Geometry check sheet. Reference: the model listing, model coordinates, mm. Round coordinates to 2 decimals unless told otherwise and drop trailing zeros. Order: outer loops, then holes, each group sorted by start corner. A loop starts at its lowest first (then second) coordinate and runs counter-clockwise, first axis right, second up.
(1) Material ranges on line 1 along Y through (x, z) = (-43, 137.3) (3 decimals); line 2 along Y through (x, z) = (-376, 136.55), recorded low to high.
(2) Sectioned sample at C-C (z = 138.15). Record the boundary of the cut face in (x, y) (3 decimals).
(3) Sectioned sample at A-A (x = -323.5). Record the boundary of the cut face in (y, z) (1 decimal).
Solid Edge part; units mm, degrees
sketch "Sketch1" plane through (0, 0, 135.9785) normal (0, 0, 1) x (1, 0, 0)
  line L0 (35.165, 9) -> (35.165, -373)
  arc A0 (35.165, -373) -> (9, -399.165) centre (9, -373) cw
  line L1 (9, -399.165) -> (-373, -399.165)
  arc A1 (-373, -399.165) -> (-399.165, -373) centre (-373, -373) cw
  line L2 (-399.165, -373) -> (-399.165, 9)
  arc A2 (-399.165, 9) -> (-373, 35.165) centre (-373, 9) cw
  line L3 (-373, 35.165) -> (9, 35.165)
  arc A3 (9, 35.165) -> (35.165, 9) centre (9, 9) cw
  line L4 (33.165, 9) -> (33.165, -373)
  line L5 (9, -397.165) -> (-373, -397.165)
  line L6 (-397.165, -373) -> (-397.165, 9)
  line L7 (-373, 33.165) -> (9, 33.165)
  arc A4 (33.165, -373) -> (9, -397.165) centre (9, -373) cw
  arc A5 (-373, -397.165) -> (-397.165, -373) centre (-373, -373) cw
  arc A6 (-397.165, 9) -> (-373, 33.165) centre (-373, 9) cw
  arc A7 (9, 33.165) -> (33.165, 9) centre (9, 9) cw
extrude "Protrusion1" add sketch "Sketch1" along normal blind 6
properties material "Polyurethene"
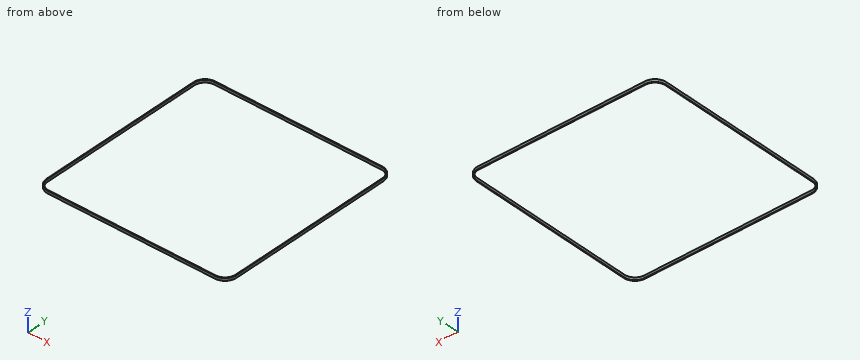
Answer below:
1. line 1: y = -399.165 to -397.165, 33.165 to 35.165
1. line 2: y = -398.99 to -396.98, 32.98 to 34.99
2. outline: (-399.165, -373) arc R26.165 ccw to (-373, -399.165) - (9, -399.165) arc R26.165 ccw to (35.165, -373) - (35.165, 9) arc R26.165 ccw to (9, 35.165) - (-373, 35.165) arc R26.165 ccw to (-399.165, 9) - close; hole (-397.165, -373) arc R24.165 ccw to (-373, -397.165) - (9, -397.165) arc R24.165 ccw to (33.165, -373) - (33.165, 9) arc R24.165 ccw to (9, 33.165) - (-373, 33.165) arc R24.165 ccw to (-397.165, 9) - close
3. outline: (-399.2, 136) - (-397.2, 136) - (-397.2, 142) - (-399.2, 142) - close; (33.2, 136) - (35.2, 136) - (35.2, 142) - (33.2, 142) - close
